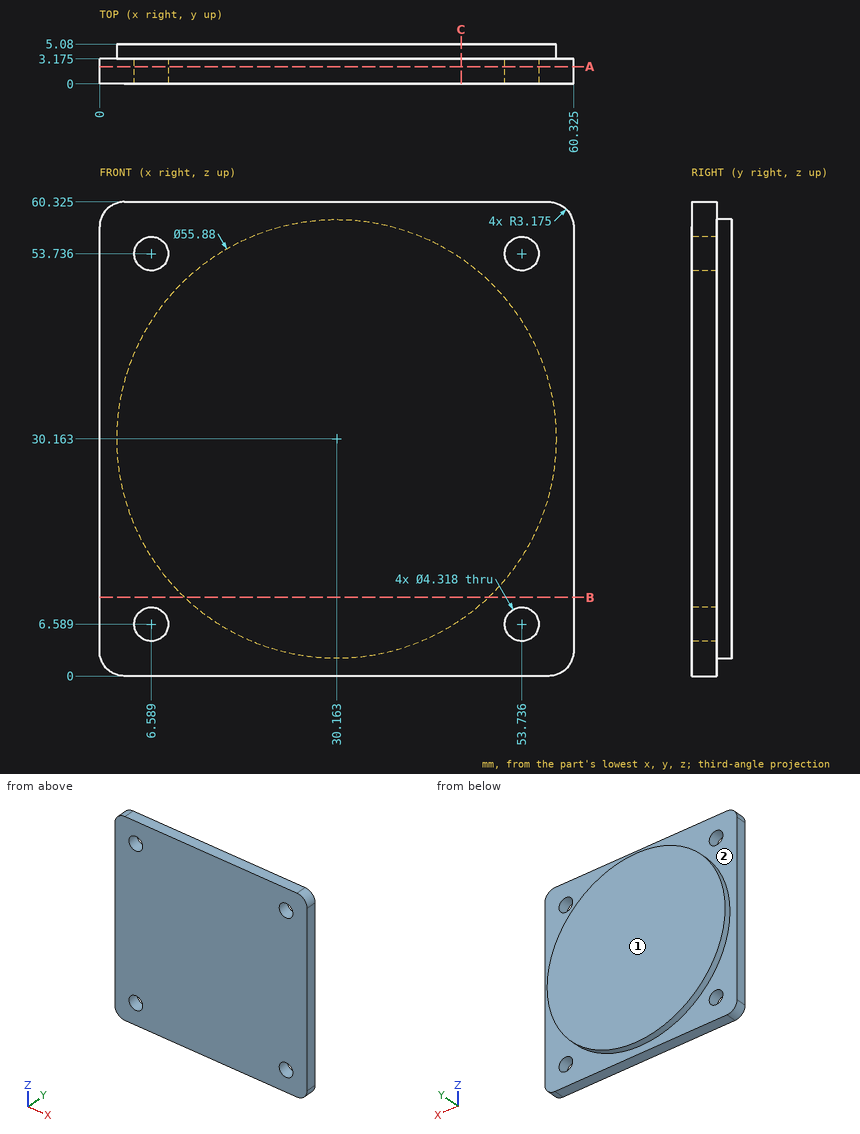
Drawing for the job (mm, zero at the part's lowest x, y, z). A direction names the side the tool comes from. Coordinates: 2 decimals unless noted, no trailing zeros. Order: outer loops, then holes, each group sorted by start corner. A loop starts at its lowest first (then second) coordinate and runs counter-clockwise, first axis right, second up. Notation, with made-up numbers: (-9.75, -6.5) -> (39.25, -6.5) arc R11 cw to (39.25, 8.5) -> close; hole circle Ø6 at (7, 41). An arc over 180 degrees is marked (long way). Answer in a Markdown table with one row per item.
1) Band-saw the part on A-A (y = 2.2). Give the number of separate pieces and of enclosed holes in the cut face, and give its area (3 significant figures).
Check values:
| item | result |
|---|---|
| separate pieces | 1 |
| enclosed holes | 4 |
| area | 3,570 mm2 |
2) Band-saw the part on C-C (x = 46). List the corners of the cut face in (y, z) (1 decimal).
Check values:
| item | result |
|---|---|
| outline | (0, 0) -> (3.2, 0) -> (3.2, 7.1) -> (5.1, 7.1) -> (5.1, 53.2) -> (3.2, 53.2) -> (3.2, 60.3) -> (0, 60.3) -> close |
3) Flat gauge pins, fed straight in: P1, Ø1.5, axis at x = 14, y = 4, coming from the -Z side; P2, Ø5, axis at x = 6.59, z = 6.59, coming from the +Y side (1 decimal). Where does each tip first touch, or does it go through?
Check values:
| item | result |
|---|---|
| P1 | z = 6.86 |
| P2 | y = 3.2 |
4) Which spindle directions (+Z, -Z, +X, -X, +Y, -Y) get a long thin tool onto all of the face, cutting with end or side? Do the marked faces 1 and 2. Say none if no direction does.
Check values:
| item | result |
|---|---|
| face 1 | +Z, -Z, +X, -X, +Y |
| face 2 | +Y |
5) Band-saw the part on B-B (z = 10). List the corners of the cut face in (x, y) (1 decimal), and give its area (3 significant figures).
Check values:
| item | result |
|---|---|
| outline | (0, 0) -> (60.3, 0) -> (60.3, 3.2) -> (49.5, 3.2) -> (49.5, 5.1) -> (10.8, 5.1) -> (10.8, 3.2) -> (0, 3.2) -> close |
| area | 265 mm2 |
6) Drill centre lines: line 1 (Y direction, x = 12, z = 54) (1 decimal); line 2 (Z direction, x = 50, y = 3.6) (1 decimal); line 3 (X direction, y = 4.75, z = 12.5) (1 decimal). Where is each one in solid material? Low to high.
Check values:
| item | result |
|---|---|
| line 1 | 0 to 3.2 |
| line 2 | 10.5 to 49.8 |
| line 3 | 8.5 to 51.8 |
